Here's the drawing with two shaded views (mm, measured from the low corner). I have some questions. Coordinates: 2 decimals unless noted, no trailing zeros. Order: outer loops, then holes, each group sorted by start corner. A loop starts at its lowest first (then second) coordinate and runs counter-clockwise, first axis right, second up. Notation, with made-up numbers: (14, -20) - (53, -20) arc R18 cw to (53, 7) - close; hole circle Ø7 at (74, 78). An arc over 180 degrees is marked (long way). Answer as CSV lines item,"result". Start each with the question number.
1. For pin 1 (5 mm diameter, centred on x = 47.5, y = 135, fed in from +Z); pin 2 (1.5 mm diameter, centred on x = 33.5, z = 14.5, fed in from +Y); pin 3 (12.5 mm diameter, centred on x = 52, z = 16.5, fed in from +Y), each with a flat end and sliding along its axis, tell me the tip position at first contact or that it passes through.
2. I want a section at D-D, the plane x = 44. List the corners of the cut face in (y, z) for me.
3. I want a section at A-A, the plane y = 135. List the corners of the cut face in (x, z) for me, and give its area (3 significant figures).
4. I want a section at C-C, the plane x = 53.5. List the corners of the cut face in (y, z) for me.
5. I need wall thicknesses on probe 1 along Y at (x, z) = (46, 27); probe 2 along Y at (x, z) = (42, 17.5). Which ranges of each line are inside material? Lowest first, please.
6. I want a section at B-B, the plane z = 21. List the corners of the cut face in (x, y) for me (1 decimal).
7. Thinking about a two-plate mould opening in Y: for the marked faces 1, 2 and 3, which applies, released by +Y, released by -Y, zero draft, split by the parting line, or undercut?
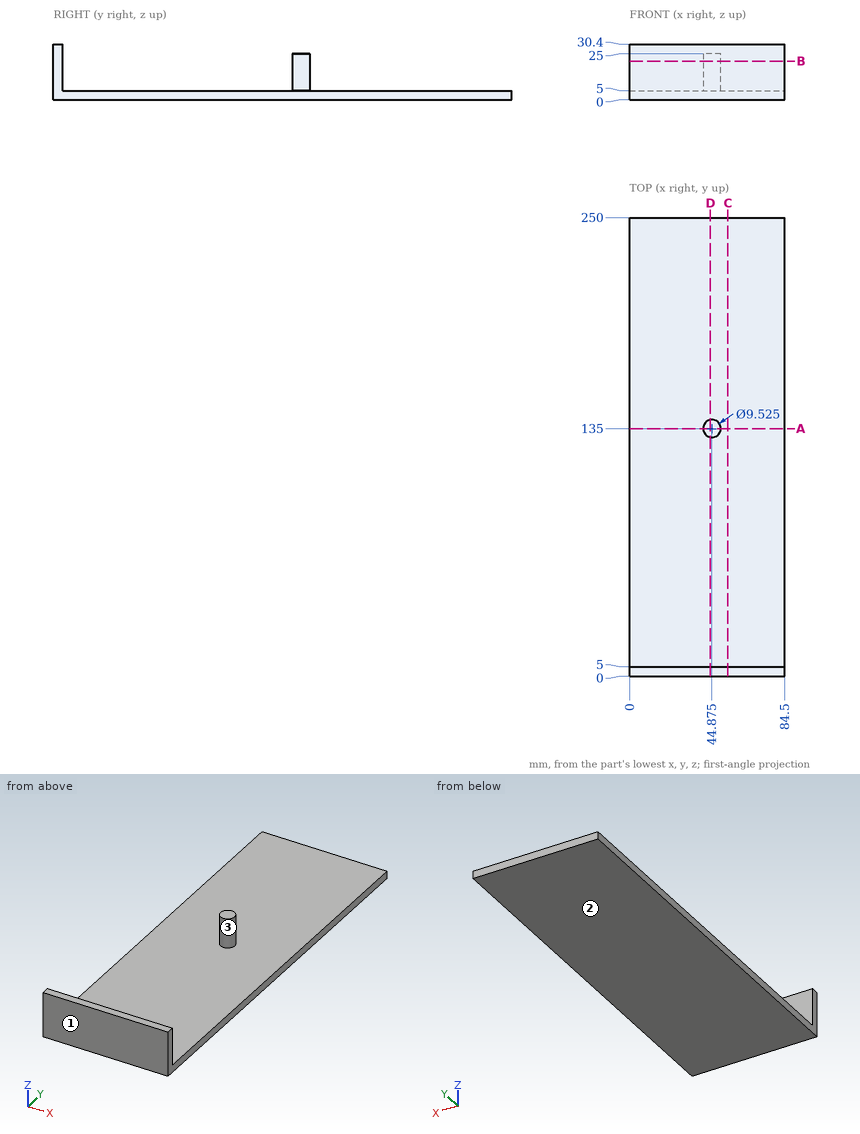
Solved:
1,pin 1,"stops at z = 25"
1,pin 2,"stops at y = 5"
1,pin 3,"stops at y = 139.68"
2,outline,"(0, 0) - (250, 0) - (250, 5) - (139.68, 5) - (139.68, 25) - (130.32, 25) - (130.32, 5) - (5, 5) - (5, 30.4) - (0, 30.4) - close"
3,outline,"(0, 0) - (84.5, 0) - (84.5, 5) - (49.64, 5) - (49.64, 25) - (40.11, 25) - (40.11, 5) - (0, 5) - close"
3,area,"613 mm2"
4,outline,"(0, 0) - (250, 0) - (250, 5) - (5, 5) - (5, 30.4) - (0, 30.4) - close"
5,probe 1,"y = 0 to 5"
5,probe 2,"y = 0 to 5, 131.2 to 138.8"
6,outline,"(0, 0) - (84.5, 0) - (84.5, 5) - (0, 5) - close; circle Ø9.5 at (44.9, 135)"
7,face 1,"released by -Y"
7,face 2,"zero draft"
7,face 3,"undercut"
